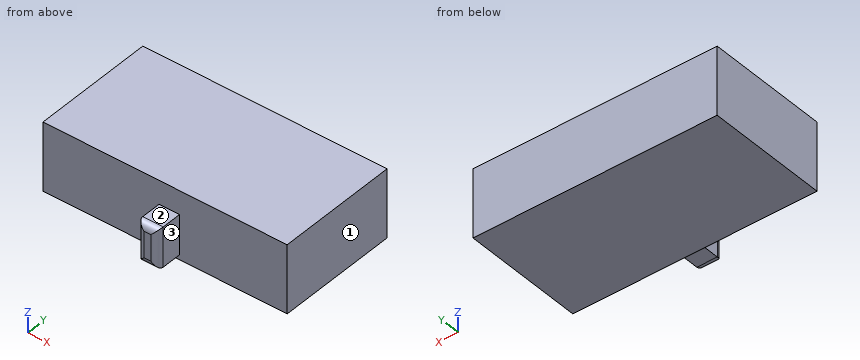
from build123d import *

# Parameters (mm, degrees)
F0_W     = 45.945797
F0_H     = 25.540538
F1_DEPTH = 91.379464
F2_W     = 7.655218
F2_H     = 14.879167
F3_DEPTH = 10.054348
F4_R     = 2.54


with BuildPart() as f1:
    # F0 (on Right) → F1 (new body)
    with BuildSketch(Plane.YZ):
        with Locations((-3.534025, 12.770269)):
            Rectangle(F0_W, F0_H)
    extrude(amount=F1_DEPTH)

    # F2 (on face) → F3 (join)
    with BuildSketch(Plane.XZ.offset(26.506923)):
        with Locations((47.253132, 9.266093)):
            Rectangle(F2_W, F2_H)
    extrude(amount=F3_DEPTH)

    # F4
    f4_edges = [f1.edges().sort_by_distance(p)[0] for p in [
        (43.425523, -36.561271, 9.266093),
        (47.253132, -36.561271, 1.82651),
        (51.080741, -36.561271, 9.266093),
        (47.253132, -36.561271, 16.705677),
    ]]
    fillet(f4_edges, radius=F4_R)


solid = f1.part
Check sheet for the modelled part. Datum: model origin and axes. Units: mm. Face numbers are marked on the shaded views. A direction names the side the tool comes from. Give positions to 0.01 mm unless a question says otherwise; leave off trailing zeros. Write each loop counter-clockwise with the first axis right and the second up, starting at its lowest first coordinate (ties: lowest second). Pieces come first, ordered by that corner, then holes. Notation, with made-up numbers: (68, 69) -> (124, 69) arc R18 ccw to (124, 82) -> close; hole circle Ø1 at (45, 10.5). An arc over 180 degrees is marked (long way). One line per item, written item: value. Start each with the question number.
Item 1: Gauge pin test, flat ends, axial feed: pin 1 (4 mm diameter, centred on y = -31, z = 9.5, fed in from -X); pin 2 (10 mm diameter, centred on x = 53.5, y = -16, fed in from -Z); pin 3 (2.5 mm diameter, centred on x = 48.5, y = -29, fed in from -Z); pin 4 (3 mm diameter, centred on x = 39.5, z = 20, fed in from -Y). Record the tip position at first contact, or that the pin passes through.
Item 2: Section check D-D on x = 28. Record the cut outline in (y, z).
Item 3: Tool access check on the marked faces 1, 2 and 3. Record the directions out of +Z, -Z, +X, -X, +Y, -Y that give a thin tool (end or side, any length) a straight path to the whole face; none if there is none.
Item 4: Section check A-A on z = 9.5. Record the cut outline in (x, y), then the cut area to 3 significant figures.
Item 5: Section check C-C on y = -31.5. Record the cut outline in (x, z).
Item 6: Material ranges on probe 1 along Y at (x, z) = (58, 3.75); probe 2 along X at (y, z) = (-29.5, 2.25); probe 3 along Z at (x, y) = (44.5, -32), recorded low to high. Write a range as from..to.
Item 7: Section check B-B on x = 45. Record the cut outline in (y, z), then the cut area to 3 significant figures.
Results list:
1. pin 1: x = 43.43
1. pin 2: z = 0
1. pin 3: z = 1.83
1. pin 4: y = -26.51
2. outline: (-26.51, 0) -> (19.44, 0) -> (19.44, 25.54) -> (-26.51, 25.54) -> close
3. face 1: +Z, -Z, +X, +Y, -Y
3. face 2: +Z, +X, -X, -Y
3. face 3: +Z, -Z, +X, -Y
4. outline: (0, -26.51) -> (43.43, -26.51) -> (43.43, -34.02) arc R2.54 ccw to (45.97, -36.56) -> (48.54, -36.56) arc R2.54 ccw to (51.08, -34.02) -> (51.08, -26.51) -> (91.38, -26.51) -> (91.38, 19.44) -> (0, 19.44) -> close
4. area: 4,270 mm²
5. outline: (43.43, 1.83) -> (51.08, 1.83) -> (51.08, 16.71) -> (43.43, 16.71) -> close
6. probe 1: -26.51..19.44
6. probe 2: 43.43..51.08
6. probe 3: 1.83..16.71
7. outline: (-36.37, 3.4) arc R2.54 ccw to (-34.02, 1.83) -> (-26.51, 1.83) -> (-26.51, 0) -> (19.44, 0) -> (19.44, 25.54) -> (-26.51, 25.54) -> (-26.51, 16.71) -> (-34.02, 16.71) arc R2.54 ccw to (-36.37, 15.13) -> close
7. area: 1,320 mm²
